Part model, mm, in its own coordinate system. A direction names the side the tool comes from. Round coordinates to 2 decimals unless told otherwise and drop trailing zeros. Loops run counter-clockwise (first coordinate to the right, second up) from the corner with the lowest first, then second, coordinate; pieces in that order, holes last.
from build123d import *

# Parameters (mm, degrees)
F0_W     = 210
F0_H     = 120
F1_DEPTH = 20
F2_R     = 40
F3_DEPTH = 50
F4_R     = 40
F5_DEPTH = 50
F6_R     = 10
F7_DEPTH = 40


with BuildPart() as f1:
    # F0 (on Right) → F1 (new body)
    with BuildSketch(Plane.YZ):
        Rectangle(F0_W, F0_H)
    extrude(amount=F1_DEPTH)

    # F2 (on face) → F3 (join)
    with BuildSketch(Plane(origin=(0, 0, 0), x_dir=(0, -1, 0), z_dir=(-1, 0, 0))):
        Circle(F2_R)
    extrude(amount=F3_DEPTH)

    # F4 (on face) → F5 (join)
    with BuildSketch(Plane.YZ.offset(20)):
        Circle(F4_R)
    extrude(amount=F5_DEPTH)

    # F6 (on face) → F7 (join)
    with BuildSketch(Plane(origin=(-50, 0, 0), x_dir=(0, -1, 0), z_dir=(-1, 0, 0))):
        Circle(F6_R)
    extrude(amount=F7_DEPTH)


solid = f1.part
1) Slice it at C-C, the plane x = 26.5. Give the cut face in (y, z), then the cut area to 3 significant figures.
Values:
outline: circle Ø80 at (0, 0)
area: 5,030 mm2
2) Slice it at D-D, the plane z = 17. Give the cut face in (x, y).
Values:
outline: (-50, -36.21) - (0, -36.21) - (0, -105) - (20, -105) - (20, -36.21) - (70, -36.21) - (70, 36.21) - (20, 36.21) - (20, 105) - (0, 105) - (0, 36.21) - (-50, 36.21) - close
3) Wall check: line 1 along X through (y, z) = (-7.5, -19); line 2 along X through (y, z) = (-93, -40); line 3 along Z through (x, y) = (-31, 22.5). Give the ranges that are in metal, low to high.
Values:
line 1: x = -50 to 70
line 2: x = 0 to 20
line 3: z = -33.07 to 33.07
4) Slice it at B-B, the plane y = 0. Give the cut face in (x, z), then the cut area to 3 significant figures.
Values:
outline: (-90, -10) - (-50, -10) - (-50, -40) - (0, -40) - (0, -60) - (20, -60) - (20, -40) - (70, -40) - (70, 40) - (20, 40) - (20, 60) - (0, 60) - (0, 40) - (-50, 40) - (-50, 10) - (-90, 10) - close
area: 11,200 mm2
5) Tool access for faces 1 (the face through (70, -1, 1)), 2 (the face through (44.65, -8.67, -39.05)), 3 (the face through (-69.72, 2.17, -9.76)): list every direction of +Z, -Z, +X, -X, +Y, -Y with a clear straight run to the whole face (end or side of a thin tool).
Values:
face 1: +Z, -Z, +X, +Y, -Y
face 2: +X
face 3: -X
6) Drop flat-ended pins along their axis: pin 1 Ø5 at (x, z) = (-10, -4.5) entering from -Y; pin 2 Ø8 at (y, z) = (-3, 34.5) entering from -X; pin 3 Ø5 at (y, z) = (-81.5, 45.5) entering from +X. Give the stop position or say it passes through.
Values:
pin 1: stops at y = -39.95
pin 2: stops at x = -50
pin 3: stops at x = 20
7) Slice it at A-A, the plane z = 0. Give the cut face in (x, y), then the cut area to 3 significant figures.
Values:
outline: (-90, -10) - (-50, -10) - (-50, -40) - (0, -40) - (0, -105) - (20, -105) - (20, -40) - (70, -40) - (70, 40) - (20, 40) - (20, 105) - (0, 105) - (0, 40) - (-50, 40) - (-50, 10) - (-90, 10) - close
area: 13,000 mm2
